Here's how the part is built. I have some questions about the finished solid (model axes, mm). Face numbers are marked on the shaded views. A direction names the side the tool comes from. Round coordinates to 2 decimals unless told otherwise and drop trailing zeros. Order: outer loops, then holes, each group sorted by start corner. A loop starts at its lowest first (then second) coordinate and runs counter-clockwise, first axis right, second up. Notation, with made-up numbers: (-15, 64) -> (33, 64) arc R21 cw to (33, 86) -> close; hole circle Ø10 at (40, -7). An arc over 180 degrees is marked (long way). Use a Markdown table: item, result. Add a question column.
from build123d import *

# Parameters (mm, degrees)
SKETCH_1_W               = 50.54
SKETCH_1_H               = 73.06
EXTRUDE_1_DEPTH          = 0.7
SKETCH_2_W               = 49.9
SKETCH_2_H               = 69
EXTRUDE_2_DEPTH          = 9
CUT_EXTRUDE_1_DEPTH      = 5
HOLE_WIZARD_M2_5_1_D     = 2.05
HOLE_WIZARD_M2_5_1_DEPTH = 4.634117865
HOLE_WIZARD_M2_5_1_TIP   = 0.615882135


with BuildPart() as part:
    # 草图1 → 凸台-拉伸1 (new body)
    with BuildSketch(Plane(origin=(0, 0, 0), x_dir=(1, 0, 0), z_dir=(0, 1, 0))):
        Rectangle(SKETCH_1_W, SKETCH_1_H)
    extrude(amount=EXTRUDE_1_DEPTH)

    # 草图2 → 凸台-拉伸2 (add)
    with BuildSketch(Plane(origin=(0, 0.7, 0), x_dir=(1, 0, 0), z_dir=(0, 1, 0))):
        with Locations((0, 0.13)):
            Rectangle(SKETCH_2_W, SKETCH_2_H)
    extrude(amount=EXTRUDE_2_DEPTH)

    # 草图6 → 切除-拉伸1 (cut)
    with BuildSketch(Plane.XY.offset(34.37)):
        with BuildLine():
            Line((-2.895, 8.7), (2.555, 8.7))
            ThreePointArc((2.555, 8.7), (4.23, 7.025), (2.555, 5.35))
            Line((2.555, 5.35), (-2.895, 5.35))
            ThreePointArc((-2.895, 5.35), (-4.57, 7.025), (-2.895, 8.7))
        make_face()
    extrude(amount=-CUT_EXTRUDE_1_DEPTH, mode=Mode.SUBTRACT)

    # M2.5 螺纹孔1
    with Locations(Plane(origin=(0, 9.7, 0), x_dir=(1, 0, 0), z_dir=(0, 1, 0))):
        with Locations((-20.55, 30.13), (20.45, 30.13), (20.45, -29.87), (-20.55, -29.87)):
            Hole(HOLE_WIZARD_M2_5_1_D / 2, depth=HOLE_WIZARD_M2_5_1_DEPTH)
            with Locations((0, 0, -(HOLE_WIZARD_M2_5_1_DEPTH + HOLE_WIZARD_M2_5_1_TIP / 2))):  # 118° drill point
                Cone(0, HOLE_WIZARD_M2_5_1_D / 2, HOLE_WIZARD_M2_5_1_TIP, mode=Mode.SUBTRACT)


solid = part.part
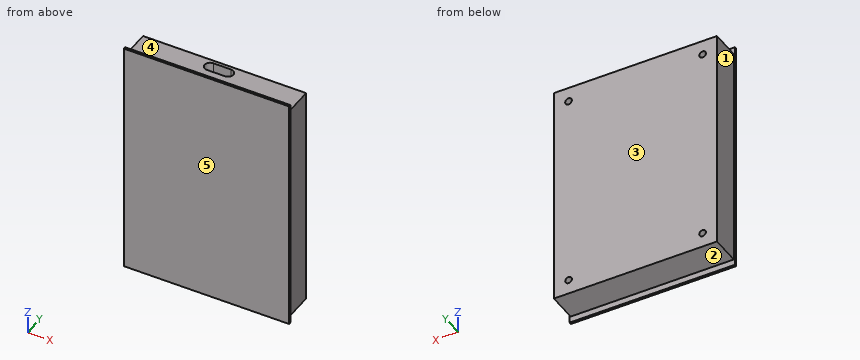
(1) On a 3-axis mill with a long thin cutter (end or side, diameter ignored), from which of +Z, -Z, +X, -X, +Y, -Y can I reach the whole of each face in a straight line? I mean the marked faces 1, 2, 3, 4 and 5. Say none if no direction works.
(2) I want a section at A-A on x = -18.5. List the corners of the cut face in (y, z) for me, and give its area (3 significant figures).
(3) I want a section at C-C on y = 2.5. List the corners of the cut face in (x, z) for me.
(4) I'm going to push flat-ended pins straight in: P1, Ø4, axis at x = 4, y = 5, coming from the -Z side; P2, Ø4.5, axis at x = 6, y = 4.5, coming from the +Z side; P3, Ø1.8, axis at x = -20.55, z = 29.87, coming from the +Y side. Where does each tip first touch, or does it pass through?
(5) Please list where these lines run through material, in increasing order: probe 1 along Z at (x, y) = (-20.55, 8.1) (3 decimals); probe 2 along X at (y, z) = (7.25, -30.13) (3 decimals); probe 3 along Z at (x, y) = (-13, 2). Write a range as from..to.
(6) I want a section at B-B on y = 6.5. List the corners of the cut face in (x, z) for me (3 decimals).
Output:
| question | item | result |
|---|---|---|
| 1 | face 1 | +Z, -Z, -X, +Y |
| 1 | face 2 | -Z, +X, -X, +Y |
| 1 | face 3 | +Z, -Z, +X, -X, +Y |
| 1 | face 4 | +Z, +X, -X, +Y |
| 1 | face 5 | +Z, -Z, +X, -X, -Y |
| 2 | outline | (0, -36.53) -> (0.7, -36.53) -> (0.7, -34.63) -> (9.7, -34.63) -> (9.7, 34.37) -> (0.7, 34.37) -> (0.7, 36.53) -> (0, 36.53) -> close |
| 2 | area | 672 mm² |
| 3 | outline | (-24.95, -34.63) -> (24.95, -34.63) -> (24.95, 34.37) -> (-24.95, 34.37) -> close |
| 4 | P1 | z = -34.63 |
| 4 | P2 | z = 34.37 |
| 4 | P3 | y = 4.99 |
| 5 | probe 1 | -34.63..-31.155, -29.105..28.845, 30.895..34.37 |
| 5 | probe 2 | -24.95..-21.575, -19.525..19.425, 21.475..24.95 |
| 5 | probe 3 | -34.63..34.37 |
| 6 | outline | (-24.95, -34.63) -> (24.95, -34.63) -> (24.95, 34.37) -> (4.146, 34.37) -> (4.146, 29.37) -> (-4.486, 29.37) -> (-4.486, 34.37) -> (-24.95, 34.37) -> close; hole circle Ø2.05 at (-20.55, -30.13); hole circle Ø2.05 at (-20.55, 29.87); hole circle Ø2.05 at (20.45, -30.13); hole circle Ø2.05 at (20.45, 29.87) |
